from build123d import *

# Parameters (mm, degrees)
F0_R     = 66.604368
F1_DEPTH = 12.7
F3_D     = 25.4
F4_D     = 38.1


with BuildPart() as f1:
    # F0 (on Front) → F1 (new body)
    with BuildSketch(Plane.XZ):
        Circle(F0_R)
    extrude(amount=F1_DEPTH)

    # F3 (through all)
    with Locations(Plane(origin=(0, 0, 0), x_dir=(1, 0, 0), z_dir=(0, 1, 0))):
        with Locations((0, 0)):
            Hole(F3_D / 2)

    # F4 (through all)
    with Locations(Plane.XZ.offset(12.7)):
        with Locations((-53.510338, 24.680197), (30.987347, 44.80923), (-24.312185, -50.30597)):
            Hole(F4_D / 2)


solid = f1.part
Model file for the job. Use its own axes, mm. Round coordinates to 2 decimals unless told otherwise and drop trailing zeros. Loops run counter-clockwise (first coordinate to the right, second up) from the corner with the lowest first, then second, coordinate; pieces in that order, holes last. Notation, with made-up numbers: M 78.25,-17.5 L 94.25,-17.5 A18 cw 94.25,-12.5 Z; hole C 22.25,85 d4. An arc over 180 degrees is marked long. One line per question, with ' | ' between items.
1) Band-saw the part on A-A (z = 0). Give the cut face in (x, y), then the cut area to 3 significant figures.
Solved:
outline: M -66.6,-12.7 L -12.7,-12.7 L -12.7,0 L -66.6,0 Z; M 12.7,-12.7 L 66.6,-12.7 L 66.6,0 L 12.7,0 Z | area: 1,370 mm²
2) Drill centre lines: line 1 along X through (y, z) = (-1.5, -0.5); line 2 along X through (y, z) = (-10.75, 34); line 3 along Z through (x, y) = (8, -5.75). Where is each one in solid material? Low to high.
Solved:
line 1: x = -66.6 to -12.69, 12.69 to 66.6 | line 2: x = -36.9 to 15.3, 46.67 to 57.27 | line 3: z = -66.12 to -9.86, 9.86 to 66.12
3) Flat gauge pins, fed straight in: pin 1 (1.5 mm diameter, centred on y = -3.5, z = 47, fed in from -X); pin 2 (4 mm diameter, centred on y = -2.5, z = -40.5, fed in from +X); pin 3 (3 mm diameter, centred on y = -1.5, z = 29.5, fed in from -X). Where does each tip first touch, or does it go through?
Solved:
pin 1: stops at x = -47.93 | pin 2: stops at x = 54.35 | pin 3: stops at x = -35.54
4) Band-saw the part on B-B (x = 0). Give the cut face in (y, z), then the cut area to 3 significant figures.
Solved:
outline: M -12.7,-66.6 L 0,-66.6 L 0,-12.7 L -12.7,-12.7 Z; M -12.7,12.7 L 0,12.7 L 0,66.6 L -12.7,66.6 Z | area: 1,370 mm²
5) Band-saw the part on D-D (z = 58.5). Give the cut face in (x, y).
Solved:
outline: M -31.84,-12.7 L 17.74,-12.7 L 17.74,0 L -31.84,0 Z
6) Band-saw the part on C-C (y = -4.5). Give the cut face in (x, z), then the cut area to 3 significant figures.
Solved:
outline: M -65.83,10.15 A66.6 ccw -43.36,-50.56 A19.05 cw long -12.67,-65.39 A66.6 ccw 50.02,43.98 A19.05 cw long 23.49,62.32 A66.6 ccw -50.45,43.48 A19.05 cw long Z; hole C 0,0 d25.4 | area: 10,700 mm²
7) Mould opens along Z. For faces 1 (the cylindrical face through (-15.89, -6.26, 64.68)), 2 (the cylindrical face through (-16.515, -6.261, -32.925)), 3 (the flat face through (14, 0, 1)) say: +Z half, -Z half, draft (parallel to the pull), parting line (faces both ways), or undercut.
Solved:
face 1: +Z half | face 2: undercut | face 3: draft
